Read the model definition and answer for the solid it produces. Units are mm, in the model's axes. Face numbers are marked on the shaded views. A direction names the side the tool comes from. Coordinates: 2 decimals unless noted, no trailing zeros. Loops run counter-clockwise (first coordinate to the right, second up) from the corner with the lowest first, then second, coordinate; pieces in that order, holes last. Notation, with made-up numbers: (50, -33) -> (103, -33) arc R19 ccw to (103, -15) -> close; hole circle Ø2 at (83.5, -34.5). An arc over 180 degrees is marked (long way). Answer as a JSON object with one key per item and string values. Group by question number.
Q1. The part is cut by section A-A on y = 3. Write down the section's boundary in (x, z), and give its area (3 significant figures).
Q2. Each of these flat-tipped pins is pushed along its axis until it touches: P1, Ø1.5, axis at x = -2.5, z = 4.5, coming from the -Y side; P2, Ø0.9, axis at x = -3, z = 4, coming from the +Y side; P3, Ø1.5, axis at y = -3.5, z = 5, coming from the +X side. Where does it stop, or does it pass through?
Q3. The part is cut by section D-D on z = 0. Write down the section's boundary in (x, y).
Q4. The part is cut by section B-B on x = 4.25. Write down the section's boundary in (y, z).
Q5. The part is cut by section C-C on z = 2.5. Write down the section's boundary in (x, y).
Q6. For the marked faces 1, 2 and 3, determine the directions among +Z, -Z, +X, -X, +Y, -Y from which every point of the face is accessible in a straight line to the end or side of a thin tool.
Q7. Straight lines are drawn through the part: line 1 along Z through (x, y) = (3, 0.75); line 2 along X through (y, z) = (0.5, 4.5); line 3 along Y through (x, z) = (-3, 3.75). For each, find the intervals that lie inside material, in ascending order. Write a range as [from, to].
from build123d import *

# Parameters (mm, degrees)
SKETCH_1_W               = 9
SKETCH_1_H               = 9
EXTRUDE_2_DEPTH          = 3
SKETCH_4_W               = 3
SKETCH_4_H               = 3
EXTRUDE_3_DEPTH          = 3
MIRROR_2_DEPTH           = 2.683281573
MIRROR_2_DRAFT           = 11.536959
MIRROR_2_2_DEPTH         = 2.683281573
MIRROR_2_2_DRAFT         = 11.536959
EXTRUDE_4_DEPTH          = 3
PATTERN_CIRCULAR_1_COUNT = 4


# Read off the part's stored shape, not the designer's step: 镜向2
with BuildPart() as part:
    # 草图1 → 凸台-拉伸2 (new, symmetric)
    with BuildSketch(Plane.XY):
        Rectangle(SKETCH_1_W, SKETCH_1_H)
    extrude(amount=EXTRUDE_2_DEPTH, both=True)

    # 草图4 → 凸台-拉伸3 (add)
    with BuildSketch(Plane.XY.offset(3)):
        Rectangle(SKETCH_4_W, SKETCH_4_H)
    extrude(amount=EXTRUDE_3_DEPTH)

    # 草图5 → 切除-放样1 section 0
    with BuildSketch(Plane.XY.offset(3), mode=Mode.PRIVATE) as loft_1_s0:
        with BuildLine():
            Line((1.5, -1.5), (4.5, -1.5))
            Line((4.5, -1.5), (4.5, -4.5))
            Line((4.5, -4.5), (1.5, -4.5))
            Line((1.5, -4.5), (1.5, -1.5))
        make_face()
    loft_1 = loft([Vertex(4.5, -4.5, -3), loft_1_s0.sketch], mode=Mode.SUBTRACT)

    # 镜向1: 切除-放样1 across plane
    add(loft_1.mirror(Plane.ZX), mode=Mode.SUBTRACT)


with BuildPart() as mirror_2_tool:
    # 镜向2 outline → 镜向2 (with draft: the straight prism first)
    with BuildSketch(Plane(origin=(-2.4, 0, 1.2), x_dir=(0.4472135954999576, 0, 0.8944271909999161), z_dir=(0.894427190999916, 0, -0.447213595499958))):
        Polygon((-4.695742753, 4.5), (2.01246118, 1.5), (2.01246118, 4.5), align=None)
    extrude(amount=-MIRROR_2_DEPTH)
    # 镜向2: the draft: its side faces are tilted about the plane it starts from
    mirror_2_sides = [mirror_2_tool.faces().sort_by_distance(p)[0] for p in [
        (-4.2, -3, 0.6),
        (-2.7, -3, 3.6),
        (-4.2, -4.5, 0.6),
    ]]
    draft(mirror_2_sides, Plane(origin=(-2.4, 0, 1.2), x_dir=(0.4472135954999576, 0, 0.8944271909999161), z_dir=(0.894427190999916, 0, -0.447213595499958)), MIRROR_2_DRAFT)


with BuildPart() as part_1:
    add(part.part)

    # 镜向2: cut by mirror_2_tool
    add(mirror_2_tool.part, mode=Mode.SUBTRACT)


with BuildPart() as mirror_2_2_tool:
    # Mirror 2 2 outline → Mirror 2 2 (with draft: the straight prism first)
    with BuildSketch(Plane(origin=(-2.4, 0, 1.2), x_dir=(0.4472135954999576, 0, 0.8944271909999161), z_dir=(0.894427190999916, 0, -0.447213595499958))):
        Polygon((2.01246118, -4.5), (2.01246118, -1.5), (-4.695742753, -4.5), align=None)
    extrude(amount=-MIRROR_2_2_DEPTH)
    # Mirror 2 2: the draft: its side faces are tilted about the plane it starts from
    mirror_2_2_sides = [mirror_2_2_tool.faces().sort_by_distance(p)[0] for p in [
        (-2.7, 3, 3.6),
        (-4.2, 3, 0.6),
        (-4.2, 4.5, 0.6),
    ]]
    draft(mirror_2_2_sides, Plane(origin=(-2.4, 0, 1.2), x_dir=(0.4472135954999576, 0, 0.8944271909999161), z_dir=(0.894427190999916, 0, -0.447213595499958)), MIRROR_2_2_DRAFT)


with BuildPart() as part_2:
    add(part_1.part)

    # Mirror 2 2: cut by mirror_2_2_tool
    add(mirror_2_2_tool.part, mode=Mode.SUBTRACT)

    # 草图7 → 凸台-拉伸4 (add)
    with BuildSketch(Plane.XZ.offset(1.5)):
        Polygon((1.5, 6), (4.5, 3), (1.5, 3), align=None)
    extrude_4 = extrude(amount=-EXTRUDE_4_DEPTH)

    # 阵列(圆周)1: 凸台-拉伸4 ×4 about axis
    pattern_circular_1_axis = Axis((0, 0, 0), (0, 0, 1))
    for i in range(1, PATTERN_CIRCULAR_1_COUNT):
        add(extrude_4.rotate(pattern_circular_1_axis, i * 360 / PATTERN_CIRCULAR_1_COUNT))


solid = part_2.part
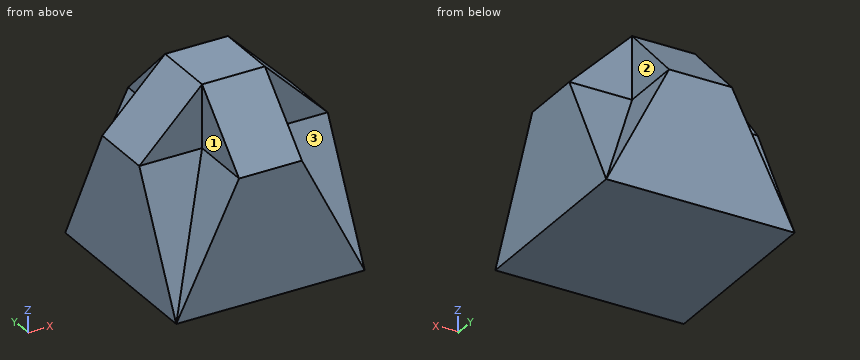
Final values:
{
 "1": {"outline": "(-4.5, -3) -> (4.5, -3) -> (4.5, 0) -> (3, 0) -> (1.5, 3) -> (1.5, 4.5) -> (-1.5, 4.5) -> (-1.5, 3) -> (-3, 0) -> (-4.5, 0) -> close", "area": "45.0 mm2"},
 "2": {"P1": "stops at y = -1.5", "P2": "stops at y = 1.5", "P3": "stops at x = 1.5"},
 "3": {"outline": "(-4.5, -3) -> (-3, -3) -> (-3, -4.5) -> (3, -4.5) -> (3, -3) -> (4.5, -3) -> (4.5, 3) -> (3, 3) -> (3, 4.5) -> (-3, 4.5) -> (-3, 3) -> (-4.5, 3) -> close"},
 "4": {"outline": "(-4.5, -3) -> (4.5, -3) -> (4.5, -2.5) -> (4.25, -2.5) -> (1.5, 3) -> (1.5, 3.25) -> (-1.5, 3.25) -> (-1.5, 3) -> (-4.25, -2.5) -> (-4.5, -2.5) -> close"},
 "5": {"outline": "(-4.5, -1.75) -> (-1.75, -1.75) -> (-1.75, -4.5) -> (1.75, -4.5) -> (1.75, -1.75) -> (4.5, -1.75) -> (4.5, 1.75) -> (1.75, 1.75) -> (1.75, 4.5) -> (-1.75, 4.5) -> (-1.75, 1.75) -> (-4.5, 1.75) -> close"},
 "6": {"face 1": "+Z, -X, -Y", "face 2": "+Z, +X, +Y", "face 3": "+Z, +X, -Y"},
 "7": {"line 1": "z = [-3, 4.5]", "line 2": "x = [-3, 3]", "line 3": "y = [-1.5, 1.5]"}
}
